```python
from build123d import *

# Parameters (mm, degrees)
SKETCH_2_R              = 12
EXTRUDE_1_DEPTH         = 8
SWEEP_3_PITCH           = 8
SURFACE_START           = -14
SURFACE_CUT_2_OUTLINE_W = 28
SURFACE_CUT_2_OUTLINE_H = 22
SURFACE_CUT_2_DEPTH     = 15.943319485


with BuildPart() as part:
    # Эскиз2 → Бобышка-Вытянуть1 (new, symmetric)
    with BuildSketch(Plane(origin=(0, 0, 0), x_dir=(1, 0, 0), z_dir=(0, 1, 0))):
        with Locations(Location((0, 0, 0), (0, 0, 270))):
            Circle(SKETCH_2_R)
    extrude(amount=EXTRUDE_1_DEPTH, both=True)

    # Вырез-По траектории3: arcs per turn and ends read off the stored shape
    # Вырез-По траектории3: the profile of Эскиз5<2> screwed along a right-hand helix through 1 turns, 14 arcs to a turn; built about Z, then put on its axis
    sweep_3_z = Axis((0, 0, 0), (0, 0, 1))
    sweep_3_corners = [(17.464, 0, 2), (2.536, 0, 5.999945545), (17.464, 0, 9.999891089)]
    with BuildLine(mode=Mode.PRIVATE) as sweep_3_profile:
        Line(sweep_3_corners[0], sweep_3_corners[1])
        Line(sweep_3_corners[1], sweep_3_corners[2])
        Line(sweep_3_corners[2], sweep_3_corners[0])
    sweep_3_cap = Face(sweep_3_profile.wire())
    sweep_3_turn_angles = [0, 12.857142857, 25.714285714, 38.571428571, 51.428571429, 64.285714286, 77.142857143, 90, 102.857142857, 115.714285714, 128.571428571, 141.428571429, 154.285714286, 167.142857143, 180, 192.857142857, 205.714285714, 218.571428571, 231.428571429, 244.285714286, 257.142857143, 270, 282.857142857, 295.714285714, 308.571428571, 321.428571429, 334.285714286, 347.142857143, 360]
    sweep_3_turn_weights = [1, 0.9749279121818236, 1, 0.9749279121818236, 1, 0.9749279121818236, 1, 0.9749279121818236, 1, 0.9749279121818236, 1, 0.9749279121818236, 1, 0.9749279121818236, 1, 0.9749279121818236, 1, 0.9749279121818236, 1, 0.9749279121818236, 1, 0.9749279121818236, 1, 0.9749279121818237, 1, 0.9749279121818236, 1, 0.9749279121818236, 1]
    sweep_3_turn_rails = [Edge.make_bspline([Vector(p[0], p[1], 0).rotate(sweep_3_z, sweep_3_turn_angles[k]) / sweep_3_turn_weights[k] + Vector(0, 0, p[2] + SWEEP_3_PITCH * sweep_3_turn_angles[k] / 360) for k in range(29)], [0, 0, 0, 1, 1, 2, 2, 3, 3, 4, 4, 5, 5, 6, 6, 7, 7, 8, 8, 9, 9, 10, 10, 11, 11, 12, 12, 13, 13, 14, 14, 14], 2, sweep_3_turn_weights) for p in sweep_3_corners]
    sweep_3_turn_sides = [Face.make_surface_from_curves(sweep_3_turn_rails[p[0]], sweep_3_turn_rails[p[1]]) for p in [(0, 1), (1, 2), (2, 0)]]
    sweep_3 = Plane(origin=(0, -8, 0), x_dir=(0, 0, -1), z_dir=(0, 1, 0)) * Solid(Shell([*sweep_3_turn_sides, sweep_3_cap, sweep_3_cap.rotate(sweep_3_z, 360).moved(Location((0, 0, SWEEP_3_PITCH * 360 / 360)))]))
    add(sweep_3, mode=Mode.SUBTRACT)

    # Surface Cut 2: read off the stored shape, not the designer's step
    # Surface Cut 2 outline → Surface Cut 2 (cut)
    with BuildSketch(Plane(origin=(0, 0, 0), x_dir=(0.8703668320896428, -0.09824022777399519, 0.48250433702211726), z_dir=(0.4924038765061049, 0.17364817766692997, -0.8528685319524428)).offset(SURFACE_START)):
        Rectangle(SURFACE_CUT_2_OUTLINE_W, SURFACE_CUT_2_OUTLINE_H)
    extrude(amount=SURFACE_CUT_2_DEPTH, mode=Mode.SUBTRACT)


solid = part.part
```
CAD build for the part. Positions are in the model's coordinates, mm. A direction names the side the tool comes from. Coordinates: 2 decimals unless noted, no trailing zeros. Write each loop counter-clockwise with the first axis right and the second up, starting at its lowest first coordinate (ties: lowest second). Pieces come first, ordered by that corner, then holes. Notation, with made-up numbers: (35, -10) -> (54, -10) arc R35 cw to (54, 29) -> close; hole circle Ø2 at (6.5, 39.25). An arc over 180 degrees is marked (long way). Use CSV: the item, a comma, the result in double quotes. Start each with the question number.
Item 1: Band-saw the part on A-A, the plane y = -5. Write the cut outline in (x, z), plus the area to 3 significant figures.
Item 2: Wall check: probe 1 along Y at (x, z) = (6, -6); probe 2 along Y at (x, z) = (9.5, -1); probe 3 along X at (y, z) = (5.5, -10.5). Give the ranges that are in metal, low to high.
Item 3: Band-saw the part on B-B, the plane y = -6.75. Write the cut outline in (x, z).
Item 4: Two-plate mould, pull along Y, no slides. Class faces 3 (the flat face through (4, -8, -6)), 4 (the flat face through (4, 8, -5)), 5 (the flat face through (0, 6, -8)): +Y half, -Y half, draft (parallel to the pull), parting line (faces both ways), or undercut.
Item 5: Tool access for faces 1 (the cylindrical face through (11.875, 7.224, -1.73)), 2 (the flat face through (0, -2, -8)): list every direction of +Z, -Z, +X, -X, +Y, -Y with a clear straight run to the whole face (end or side of a thin tool).
Item 6: Drop flat-ended pins along their axis: P1, Ø5.5, axis at y = -2.5, z = -6.5, coming from the -X side; P2, Ø2, axis at y = 5.5, z = 3.5, coming from the +X side; P3, Ø3, axis at x = -2.5, y = 4.5, coming from the +Z side. Give the stop position or say it passes through.
Response values:
1,outline,"(-8.67, -8.3) arc R12 ccw to (11.52, 3.36) -> close"
1,area,"158 mm2"
2,probe 1,"y = -8 to 3.4, 6.59 to 8"
2,probe 2,"y = -8 to 2.25, 6.01 to 8"
2,probe 3,"x = -5.81 to 0"
3,outline,"(-8.44, -8.53) arc R12 ccw to (11.61, 3.05) -> close"
4,face 3,"-Y half"
4,face 4,"+Y half"
4,face 5,"undercut"
5,face 1,"+X, +Y, -Y"
5,face 2,"-Z"
6,P1,"stops at x = -8.85"
6,P2,"stops at x = 11.66"
6,P3,"stops at z = -1.89"
